from build123d import *

# Parameters (mm, degrees)
SZKIC1_W                        = 5
SZKIC1_H                        = 29
WYTNIJ_WYCI_GNI_CIE1_DEPTH      = 15
WYTNIJ_WYCI_GNI_CIE1_DEPTH_BACK = 15
SZKIC3_R                        = 11
WYTNIJ_WYCI_GNI_CIE2_DEPTH      = 6
WYTNIJ_WYCI_GNI_CIE2_DEPTH_BACK = 6
SFAZOWANIE1_SIZE                = 1.45


with BuildPart() as part:
    # Szkic1 → Obrót1 (revolve)
    with BuildSketch(Plane(origin=(0, 0, 0), x_dir=(1, 0, 0), z_dir=(0, 1, 0))):
        with BuildLine():
            Line((0, 14), (0, -19))
            Line((0, -19), (5, -19))
            Line((5, -19), (12.037712352, -7.147970434))
            ThreePointArc((12.037712352, -7.147970434), (12.166996056, 6.925619609), (0, 14))
        make_face()
        with Locations((2.5, -33.5)):
            Rectangle(SZKIC1_W, SZKIC1_H)
    revolve(axis=Axis((0, 0, -26.043516498), (0, 0, 1)))

    # Szkic2 → Wytnij-wyciągnięcie1 (cut, two sides)
    with BuildSketch(Plane(origin=(0, 0, 0), x_dir=(0, 0, -1), z_dir=(1, 0, 0))) as wytnij_wyci_gni_cie1_sk:
        with BuildLine():
            Line((-19, 5), (13.076696831, 5))
            ThreePointArc((13.076696831, 5), (4.601064873, 13.222337238), (-7.147970434, 12.037712352))
            Line((-7.147970434, 12.037712352), (-19, 5))
        make_face()
        with BuildLine():
            Line((-19, -5), (13.076696831, -5))
            ThreePointArc((13.076696831, -5), (4.601064873, -13.222337238), (-7.147970434, -12.037712352))
            Line((-7.147970434, -12.037712352), (-19, -5))
        make_face()
    extrude(amount=WYTNIJ_WYCI_GNI_CIE1_DEPTH, mode=Mode.SUBTRACT)
    extrude(wytnij_wyci_gni_cie1_sk.sketch, amount=-WYTNIJ_WYCI_GNI_CIE1_DEPTH_BACK, mode=Mode.SUBTRACT)

    # Szkic3 → Wytnij-wyciągnięcie2 (cut, two sides)
    with BuildSketch(Plane(origin=(0, 0, 0), x_dir=(1, 0, 0), z_dir=(0, 1, 0))) as wytnij_wyci_gni_cie2_sk:
        Circle(SZKIC3_R)
    extrude(amount=WYTNIJ_WYCI_GNI_CIE2_DEPTH, mode=Mode.SUBTRACT)
    extrude(wytnij_wyci_gni_cie2_sk.sketch, amount=-WYTNIJ_WYCI_GNI_CIE2_DEPTH_BACK, mode=Mode.SUBTRACT)

    # Sfazowanie1
    sfazowanie1_edges = [part.edges().sort_by_distance(p)[0] for p in [
        (-5, 0, 48),
    ]]
    chamfer(sfazowanie1_edges, length=SFAZOWANIE1_SIZE)


solid = part.part
Here's how the part is built. I have some questions about the finished solid (model axes, mm). A direction names the side the tool comes from. Give positions to 0.01 mm unless a question says otherwise; leave off trailing zeros. Loops run counter-clockwise (first coordinate to the right, second up) from the corner with the lowest first, then second, coordinate; pieces in that order, holes last. Notation, with made-up numbers: (6, 35.25) -> (23, 35.25) arc R18 ccw to (23, 63.25) -> close; hole circle Ø1 at (73.5, -21.75). An arc over 180 degrees is marked (long way). One line per item, written item: value.
Q1. On a 3-axis mill with a long thin cutter (end or side, diameter ignored), from which of +Z, -Z, +X, -X, +Y, -Y can I reach the whole of each face in a straight line? I mean faces 4 (the face through (-2.38, 0.07, 10.74)), 5 (the face through (-1.08, -4.88, 32.58)). Say none if no direction works.
Answers follow:
face 4: +Y, -Y
face 5: +Z
Q2. Suppose I cut it at A-A on z = 0. Please give me the cut outline in (x, y), then the cut area to 3 significant figures.
Answers follow:
outline: (-13.08, -5) -> (-11, -5) -> (-11, 5) -> (-13.08, 5) arc R14 ccw to start; (11, -5) -> (13.08, -5) arc R14 ccw to (13.08, 5) -> (11, 5) -> close
area: 53.9 mm^2
Q3. If I drill on line 1 along Z through (x, y) = (0, 0.5); line 2 along X through (y, z) = (0, 0); line 3 along X through (y, z) = (0, 21.5), over which ranges is the centre line in solid material (lowest first)?
Answers follow:
line 1: -13.99 to -11, 11 to 48
line 2: -14 to -11, 11 to 14
line 3: -5 to 5
Q4. Suppose I cut it at B-B on y = 0. Please give me the cut outline in (x, z).
Answers follow:
outline: (-12.04, 7.15) arc R14 ccw (long way) to (12.04, 7.15) -> (5, 19) -> (5, 46.55) -> (3.55, 48) -> (-3.55, 48) -> (-5, 46.55) -> (-5, 19) -> close; hole circle Ø22 at (0, 0)
Q5. We'd pull the mould along Y, two halves only. Please class faces 1 (the face through (-0.1, 5, 11.4)), 2 (the face through (0, 0, 48)), 3 (the face through (-0.1, -5, 11.4)): pulls with the +Y half, pulls with the -Y half, needs draft (parallel to the pull), parting line crosses it, or undercut.
Answers follow:
face 1: pulls with the +Y half
face 2: needs draft
face 3: pulls with the -Y half
Q6. I'm going to push flat-ended pins straight in: pin 1 Ø4 at (y, z) = (-2, 7) entering from -X; pin 2 Ø3 at (x, z) = (10, 16) entering from -Y; pin 3 Ø1.5 at (y, z) = (2.5, 5) entering from -X; pin 4 Ø4 at (x, y) = (-5.5, 3.5) entering from +Z. Where does each tip first touch, or does it pass through?
Answers follow:
pin 1: x = -12.97
pin 2: through
pin 3: x = -13.14
pin 4: z = 47.03
Q7. Suppose I cut it at C-C on z = 30. Please give me the cut outline in (x, y).
Answers follow:
outline: circle Ø10 at (0, 0)
